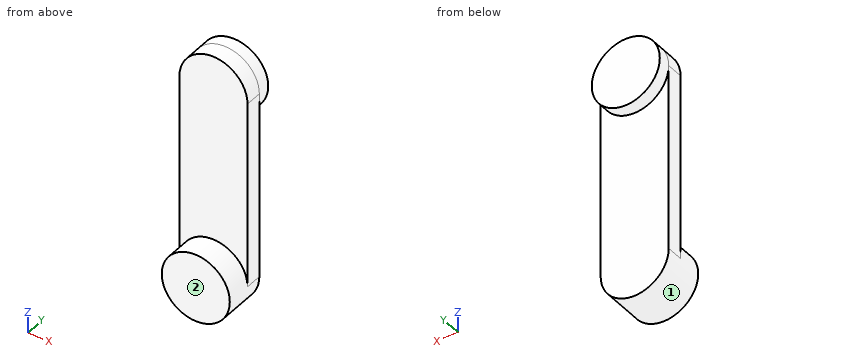
from build123d import *

# Parameters (mm, degrees)
F1_DEPTH = 3.175
F2_R     = 6.35
F3_DEPTH = 2.4
F4_R     = 6.35
F5_DEPTH = 4.7625


with BuildPart() as f1:
    # F0 (on Front) → F1 (new body)
    with BuildSketch(Plane.XZ):
        with BuildLine():
            Line((-6.35, 0), (-6.35, -34.925))
            ThreePointArc((-6.35, -34.925), (0, -41.275), (6.35, -34.925))
            Line((6.35, -34.925), (6.35, 0))
            ThreePointArc((6.35, 0), (0, 6.35), (-6.35, 0))
        make_face()
    extrude(amount=F1_DEPTH)

    # F2 (on face) → F3 (join)
    with BuildSketch(Plane(origin=(0, 0, 0), x_dir=(-1, 0, 0), z_dir=(0, 1, 0))):
        Circle(F2_R)
    extrude(amount=F3_DEPTH)

    # F4 (on face) → F5 (join)
    with BuildSketch(Plane.XZ.offset(3.175)):
        with Locations((0, -34.925)):
            Circle(F4_R)
    extrude(amount=F5_DEPTH)


solid = f1.part
Verification items for the finished model (mm, model axes). Face numbers are marked on the shaded views. A direction names the side the tool comes from. Round coordinates to 2 decimals unless told otherwise and drop trailing zeros. Loops run counter-clockwise (first coordinate to the right, second up) from the corner with the lowest first, then second, coordinate; pieces in that order, holes last. Notation, with made-up numbers: (80, 13.5) - (132, 13.5) arc R26 cw to (132, 45.5) - close; hole circle Ø4 at (89.25, 10.5). An arc over 180 degrees is marked (long way). Use a Markdown table: item, result. Add a question column.
1. Section check C-C, the plane y = -1.5. Record the boundary of the cut face in (x, z) (3 decimals), plus the area to 3 significant figures.
2. Section check A-A, the plane x = -4. Record the boundary of the cut face in (y, z) (1 decimal).
3. Access from +Z, -Z, +X, -X, +Y, -Y to the whole of each face (thin tool, end or side, straight path). Record for the marked faces 1 and 2.
4. Thickness scan on probe 1 along Y at (x, z) = (2, -31); probe 2 along Y at (x, z) = (-5, 3.5) (3 decimals); probe 3 along Z at (x, y) = (0, -3.5) (3 decimals). Record the ranges inside material, lowest first. Write a range as [from, to].
5. Gauge pin test, flat ends, axial feed: pin 1 (4 mm diameter, centred on x = -1.5, z = -19, fed in from +Y); pin 2 (1.5 mm diameter, centred on y = -1, z = -36.5, fed in from +X). Record the tip position at first contact, or that the pin passes through.
6. Section check D-D, the plane y = 1.5. Record the boundary of the cut face in (x, z).
7. Section check B-B, the plane z = -5. Record the boundary of the cut face in (x, y) (3 decimals), plus the area to 3 significant figures.
Checks:
| question | item | result |
|---|---|---|
| 1 | outline | (-6.35, -34.925) arc R6.35 ccw to (6.35, -34.925) - (6.35, 0) arc R6.35 ccw to (-6.35, 0) - close |
| 1 | area | 570 mm^2 |
| 2 | outline | (-7.9, -39.9) - (0, -39.9) - (0, -4.9) - (2.4, -4.9) - (2.4, 4.9) - (-3.2, 4.9) - (-3.2, -30) - (-7.9, -30) - close |
| 3 | face 1 | -Y |
| 3 | face 2 | +Z, -Z, +X, -X, -Y |
| 4 | probe 1 | y = [-7.94, 0] |
| 4 | probe 2 | y = [-3.175, 2.4] |
| 4 | probe 3 | z = [-41.275, -28.575] |
| 5 | pin 1 | stops at y = 0 |
| 5 | pin 2 | stops at x = 6.3 |
| 6 | outline | circle Ø12.7 at (0, 0) |
| 7 | outline | (-6.35, -3.175) - (6.35, -3.175) - (6.35, 0) - (3.914, 0) - (3.914, 2.4) - (-3.914, 2.4) - (-3.914, 0) - (-6.35, 0) - close |
| 7 | area | 59.1 mm^2 |
